Check sheet for the drawn part. Datum: minimum x, y, z corner. Units: mm. A direction names the side the tool comes from. Give positions to 0.01 mm unless a question says otherwise; leave off trailing zeros. Order: outer loops, then holes, each group sorted by start corner. A loop starts at its lowest first (then second) coordinate and runs counter-clockwise, first axis right, second up.
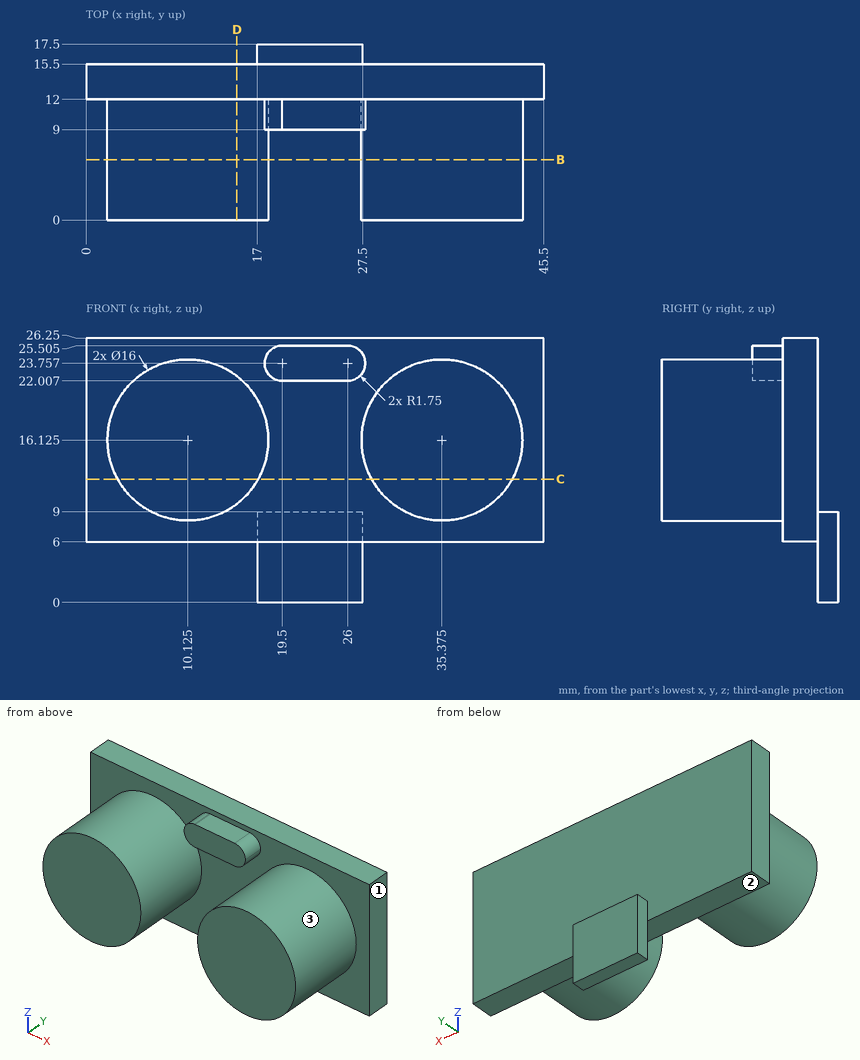
(1) Set-up check for the marked faces 1, 2 and 3: record each of +Z, -Z, +X, -X, +Y, -Y from which the full face is reachable in a straight line by a thin tool's end or side.
Solved:
face 1: +Z, -Z, +X, +Y, -Y
face 2: -Z, +X, -X, -Y
face 3: -Y
(2) Scan lines: line 1 (Y direction, x = 36.5, z = 8); line 2 (Z direction, x = 39, y = 13); line 3 (Z direction, x = 10.5, y = 3.5). Record each from-to range of solid material in increasing order.
Solved:
line 1: y = 12 to 15.5
line 2: z = 6 to 26.25
line 3: z = 8.13 to 24.12
(3) Section check C-C, the plane z = 12.25. Enter the section's corners in (x, y).
Solved:
outline: (0, 12) - (3.13, 12) - (3.13, 0) - (17.12, 0) - (17.12, 12) - (28.38, 12) - (28.38, 0) - (42.37, 0) - (42.37, 12) - (45.5, 12) - (45.5, 15.5) - (0, 15.5) - close
(4) Section check D-D, the plane x = 15. Enter the section's corners in (y, z), then the cut area to 3 significant figures.
Solved:
outline: (0, 9.78) - (12, 9.78) - (12, 6) - (15.5, 6) - (15.5, 26.25) - (12, 26.25) - (12, 22.47) - (0, 22.47) - close
area: 223 mm2
(5) Section check B-B, the plane y = 6. Enter the section's corners in (x, z) (1 decimal).
Solved:
outline: circle Ø16 at (10.1, 16.1); circle Ø16 at (35.4, 16.1)
(6) Go/stop test with flat-tipped pins: pin 1 (10 mm diameter, centred on x = 32, z = 20.5, fed in from +Y); pin 2 (1.8 mm diameter, centred on x = 22.5, y = 14.5, fed in from -Z); pin 3 (5 mm diameter, centred on x = 23, z = 2, fed in from -Y). Record where each tip stops, or that it passes through.
Solved:
pin 1: stops at y = 15.5
pin 2: stops at z = 6
pin 3: stops at y = 15.5
